from build123d import *

# Parameters (mm, degrees)
F0_W     = 84
F0_H     = 100
F1_DEPTH = 2
F2_W     = 2
F2_H     = 24
F3_DEPTH = 80
F4_W     = 84
F4_H     = 24
F5_DEPTH = 2
F7_D     = 2
F7_DEPTH = 2.001
F9_D     = 2


with BuildPart() as f1:
    # F0 (on Top) → F1 (new body)
    with BuildSketch(Plane.XY):
        with Locations((42, -50)):
            Rectangle(F0_W, F0_H)
    extrude(amount=F1_DEPTH)

    # F2 (on face) → F3 (join)
    with BuildSketch(Plane.XY.offset(2)):
        with Locations((1, -35)):
            Rectangle(F2_W, F2_H)
        with Locations((83, -35)):
            Rectangle(F2_W, F2_H)
    extrude(amount=F3_DEPTH)

    # F4 (on face) → F5 (join)
    with BuildSketch(Plane.XY.offset(82)):
        with Locations((42, -35)):
            Rectangle(F4_W, F4_H)
    extrude(amount=F5_DEPTH)

    # F7 (through all, one way)
    with BuildSketch(Plane.XY.offset(2)):
        with Locations((34, -37), (50, -37), (50, -63), (34, -63)):
            Circle(F7_D / 2)
    extrude(amount=-F7_DEPTH, mode=Mode.SUBTRACT)

    # F9 (through all)
    with Locations(Plane.YZ.offset(84)):
        with Locations((-35, 77), (-35, 67)):
            Hole(F9_D / 2)


solid = f1.part
CAD build for the part. Positions are in the model's coordinates, mm. A direction names the side the tool comes from. Round coordinates to 2 decimals unless told otherwise and drop trailing zeros. Write each loop counter-clockwise with the first axis right and the second up, starting at its lowest first coordinate (ties: lowest second). Pieces come first, ordered by that corner, then holes. Notation, with made-up numbers: M 22,-23.75 L 27,-23.75 A13 cw 27,-7.75 Z; hole C 8.5,-31 d8. An arc over 180 degrees is marked long. Put each result on its own line as item: value. Start each with the question number.
1) Saw through at A-A, the plane x = 8.5. Write the cut outline in (y, z), and give its area (3 significant figures).
2) 3-axis set-ups, long thin cutter, end or side, ignore diameter. For faces 1 (the flat face through (41.8, -47, 82.3)), 2 (the flat face through (41.8, -23, 82.3)), 3 (the flat face through (82, -35, 41)), 4 (the flat face through (84, -39, 36)): which of +Z, -Z, +X, -X, +Y, -Y reach the whole face in a straight line?
3) Pin check, flat tips, straight feed: pin 1 Ø12 at (x, y) = (65.5, -20.5) entering from -Z; pin 2 Ø4 at (x, y) = (73, -81) entering from +Z; pin 3 Ø1.6 at (y, z) = (-35, 77) entering from -X. Stop position of each tip, or through.
4) Drill centre lines: probe 1 along Z at (x, y) = (1.15, -35); probe 2 along Z at (x, y) = (27, -32.5); probe 3 along Y at (x, z) = (1.25, 67). Where is each one in solid material? Low to high. Write a range as [from, to].
5) Pull direction Z, two halves, no side cores. Call faces 5 (the flat face through (41, -35, 82)), 6 (the flat face through (41, -35, 84)), 7 (the flat face through (41, -49, 0)), 8 (the flat face through (2, -35, 41)): pulls with the +Z half, pulls with the -Z half, needs draft (parallel to the pull), parting line crosses it, or undercut.
6) Saw through at B-B, the plane z = 44. Write the cut outline in (x, y).
7) Saw through at C-C, the plane y = -51. Write the cut outline in (x, z).
Resolved:
1. outline: M -100,0 L 0,0 L 0,2 L -100,2 Z; M -47,82 L -23,82 L -23,84 L -47,84 Z
1. area: 248 mm²
2. face 1: +Z, +X, -X, -Y
2. face 2: +Z, +X, -X, +Y
2. face 3: +Y, -Y
2. face 4: +Z, -Z, +X, +Y, -Y
3. pin 1: z = 0
3. pin 2: z = 2
3. pin 3: through
4. probe 1: [0, 66], [68, 76], [78, 84]
4. probe 2: [0, 2], [82, 84]
4. probe 3: [-47, -36], [-34, -23]
5. face 5: undercut
5. face 6: pulls with the +Z half
5. face 7: pulls with the -Z half
5. face 8: undercut
6. outline: M 0,-47 L 2,-47 L 2,-23 L 0,-23 Z; M 82,-47 L 84,-47 L 84,-23 L 82,-23 Z
7. outline: M 0,0 L 84,0 L 84,2 L 0,2 Z
